from build123d import *

# Parameters (mm, degrees)
SKETCH1_W               = 48.26
SKETCH1_H               = 63.5
BOSS_EXTRUDE1_DEPTH     = 1
SKETCH3_R               = 1.143
BOSS_EXTRUDE2_DEPTH     = 3
SKETCH4_R               = 2.524
SKETCH4_R_2             = 4.064
BOSS_EXTRUDE3_DEPTH     = 1
CUT_EXTRUDE1_DEPTH      = 80.814018819
CUT_EXTRUDE1_DEPTH_BACK = 80.814018819
SKETCH2_R               = 3.175
SKETCH2_R_2             = 1.524


with BuildPart() as part:
    # Sketch1 → Boss-Extrude1 (new body)
    with BuildSketch(Plane(origin=(0, -11.34264997, 0), x_dir=(1, 0, 0), z_dir=(0, 1, 0))):
        with Locations((24.13, -31.75)):
            Rectangle(SKETCH1_W, SKETCH1_H)
    extrude(amount=BOSS_EXTRUDE1_DEPTH)

    # Sketch3 → Boss-Extrude2 (add)
    with BuildSketch(Plane.XZ.offset(11.34264997)):
        with Locations(Location((5.0673, 58.34634, 0), (0, 0, 90))):
            Circle(SKETCH3_R)
        with Locations(Location((27.31008, 5.72008, 0), (0, 0, 90))):
            Circle(SKETCH3_R)
    extrude(amount=BOSS_EXTRUDE2_DEPTH)

    # Sketch4 → Boss-Extrude3 (add)
    with BuildSketch(Plane.XZ.offset(11.34264997)):
        with Locations(Location((5.0673, 58.34634, 0), (0, 0, 90))):
            Circle(SKETCH4_R)
        with Locations(Location((37.75456, 19.90598, 0), (0, 0, 90))):
            Circle(SKETCH4_R_2)
        with Locations(Location((36.9062, 11.4046, 0), (0, 0, 90))):
            Circle(SKETCH4_R_2)
        with Locations(Location((27.31008, 5.72008, 0), (0, 0, 90))):
            Circle(SKETCH4_R)
    extrude(amount=BOSS_EXTRUDE3_DEPTH)

    # Sketch2 → Cut-Extrude1 (cut, two sides: drawn at the far end of the back side and taken through both)
    with BuildSketch(Plane.XZ.offset(11.34264997).offset(-CUT_EXTRUDE1_DEPTH_BACK)):
        with Locations(Location((37.75456, 19.90598, 0), (0, 0, 270))):
            Circle(SKETCH2_R)
        with Locations(Location((36.9062, 11.4046, 0), (0, 0, 270))):
            Circle(SKETCH2_R)
        with Locations(Location((19.6723, 19.02714, 0), (0, 0, 270))):
            Circle(SKETCH2_R_2)
    extrude(amount=CUT_EXTRUDE1_DEPTH + CUT_EXTRUDE1_DEPTH_BACK, mode=Mode.SUBTRACT)


solid = part.part
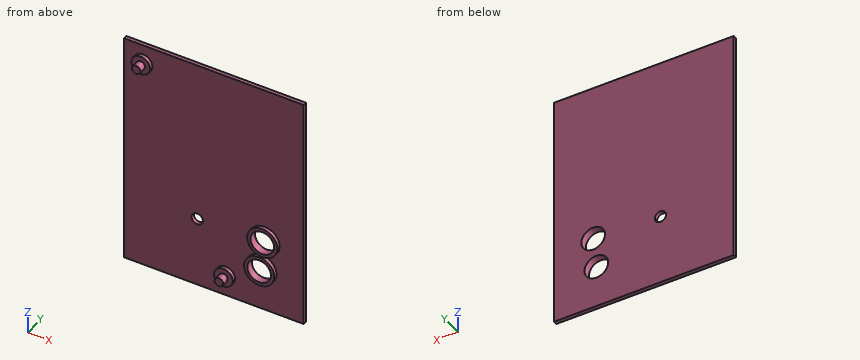
Check sheet for the modelled part. Datum: model origin and axes. Units: mm. Give positions to 0.01 mm unless a question says otherwise; leave off trailing zeros. Write each loop counter-clockwise with the first axis right and the second up, starting at its lowest first coordinate (ties: lowest second). Pieces come first, ordered by that corner, then holes. Notation, with made-up numbers: M 4,33.25 L 38,33.25 A14 ccw 38,48.25 Z; hole C 75,89 d2. An arc over 180 degrees is marked long. Use one line per item in the form item = value.
(1) Section check D-D on z = 40. Record the boundary of the cut face in (x, y).
Answer block:
outline = M 0,-11.34 L 48.26,-11.34 L 48.26,-10.34 L 0,-10.34 Z
(2) Section check B-B on y = -13.4. Record the boundary of the cut face in (x, z), plus the area to 3 significant figures.
Answer block:
outline = C 5.07,58.35 d2.29; C 27.31,5.72 d2.29
area = 8.21 mm2
(3) Section check C-C on x = 12.5. Record the boundary of the cut face in (y, z).
Answer block:
outline = M -11.34,0 L -10.34,0 L -10.34,63.5 L -11.34,63.5 Z
(4) Section check A-A on z = 10.5. Record the boundary of the cut face in (x, y).
Answer block:
outline = M 0,-11.34 L 32.94,-11.34 L 32.94,-12.34 L 33.86,-12.34 L 33.86,-10.34 L 0,-10.34 Z; M 39.95,-12.34 L 40.87,-12.34 L 40.87,-11.34 L 48.26,-11.34 L 48.26,-10.34 L 39.95,-10.34 Z
(5) Depth check by flat-ended pin: P1, Ø10, axis at x = 36.91, z = 11.4, coming from the -Y side; P2, Ø2.5, axis at x = 19.67, z = 19.03, coming from the -Y side; P3, Ø2.5, axis at x = 28.5, z = 5.5, coming from the -Y side; P4, Ø3, axis at x = 15.5, z = 42, coming from the -Y side. Enter the tip coordinate at first touch or a pass-through.
Answer block:
P1 = -12.34
P2 = through
P3 = -14.34
P4 = -11.34
(6) Material ranges on line 1 along Z through (x, y) = (36, -12.25); line 2 along Y through (x, z) = (5, 38); line 3 along Z through (x, y) = (36.5, -11.1), recorded low to high.
Answer block:
line_1 = 7.44 to 8.36, 14.45 to 15.37, 16.24 to 17.26, 22.55 to 23.57
line_2 = -11.34 to -10.34
line_3 = 0 to 8.26, 14.55 to 16.99, 22.82 to 63.5
